Could you check a few things on this model? Use its own coordinates, in mm. Face numbers are marked on the shaded views. A direction names the side the tool comes from. Coordinates: 2 decimals unless noted, no trailing zeros. Loops run counter-clockwise (first coordinate to the right, second up) from the corner with the lowest first, then second, coordinate; pieces in that order, holes last.
1) Thinking about a two-plate mould opening in X: for the marked faces 1, 2 and 3, which applies, released by +X, released by -X, zero draft, split by the parting line, or undercut?
2) Imagine slicing it at B-B on x = 0. Please give me the cut outline in (y, z) (3 decimals), plus the area to 3 significant figures.
3) Imagine slicing it at D-D on z = -2.75. Please give me the cut outline in (x, y) (3 decimals).
4) Imagine slicing it at C-C on y = 7. Please give me the cut outline in (x, z), plus the area to 3 significant figures.
5) For the marked faces 4 and 5, which set-ups out of +Z, -Z, +X, -X, +Y, -Y let a thin tool reach every point of the face, with its end or its side?
6) If I drill on line 1 along Y through (x, z) = (0, -8.75) (3 decimals); line 2 along X through (y, z) = (8.5, -3); line 3 along Y through (x, z) = (1, -2.5), over which ranges is the centre line in solid material (lowest first)?
7) Will these pins go through, and if not, where does the flat tip stop? P1, Ø11.5, axis at x = 0, y = 0, coming from the -Z side; P2, Ø3, axis at y = 6.5, z = -3.5, coming from the -X side; P3, Ø2, axis at y = 5.5, z = -6, coming from the +X side; P4, Ø6, axis at y = 4.5, z = -6, coming from the +X side.
8) Imagine slicing it at A-A on y = 0. Please give me the cut outline in (x, z) (3 decimals).
```python
from build123d import *

# Parameters (mm, degrees)
CROQUIS1_W            = 14.288
CROQUIS1_H            = 15.875
CORTAR_EXTRUIR1_REACH = 28.612
CROQUIS2_R            = 9.525
CROQUIS3_W            = 3.96875
CROQUIS3_H            = 15.875


with BuildPart() as part:
    # Croquis1 → Revolución1 (revolve)
    with BuildSketch(Plane(origin=(0, 0, 0), x_dir=(0, 0, -1), z_dir=(1, 0, 0)), mode=Mode.PRIVATE) as revoluci_n1_sk:
        with Locations((7.144, 7.9375)):
            Rectangle(CROQUIS1_W, CROQUIS1_H)
    revolve(revoluci_n1_sk.sketch.rotate(Axis((0, 0, 0), (0, 0, -1)), 90), axis=Axis((0, 0, 0), (0, 0, -1)))

    # Croquis2 → Cortar-Extruir1 (cut, up to next)
    with BuildSketch(Plane.XY, mode=Mode.PRIVATE) as cortar_extruir1_sk1:
        Circle(CROQUIS2_R)
    cortar_extruir1_tool1 = extrude(cortar_extruir1_sk1.sketch, amount=-CORTAR_EXTRUIR1_REACH, mode=Mode.PRIVATE) & part.part
    add(cortar_extruir1_tool1.solids().sort_by_distance((0, 0, 0))[0], mode=Mode.SUBTRACT)

    # Croquis3 → Taladro roscado 1/8-27 NPSM1 (revolve, cut)
    with BuildSketch(Plane(origin=(15.875, 0, -7.144), x_dir=(0, 0, -1), z_dir=(0, 1, 0))):
        with Locations((1.984375, 7.9375)):
            Rectangle(CROQUIS3_W, CROQUIS3_H)
    revolve(axis=Axis((22.225, 0, -7.144), (-1, 0, 0)), mode=Mode.SUBTRACT)


solid = part.part
```
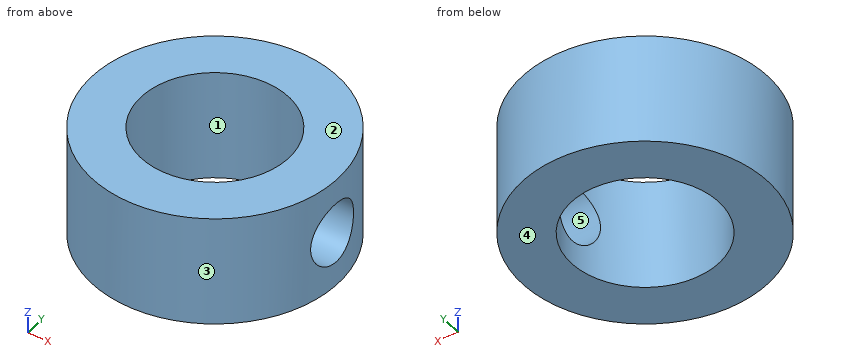
Filled in:
1. face 1: undercut
1. face 2: zero draft
1. face 3: split by the parting line
2. outline: (-15.875, -14.288) - (-9.525, -14.288) - (-9.525, 0) - (-15.875, 0) - close; (9.525, -14.288) - (15.875, -14.288) - (15.875, 0) - (9.525, 0) - close
2. area: 181 mm2
3. outline: circle Ø31.75 at (0, 0); hole circle Ø19.05 at (0, 0)
4. outline: (-14.25, -14.29) - (-6.46, -14.29) - (-6.46, 0) - (-14.25, 0) - close; (6.46, -14.29) - (14.25, -14.29) - (14.25, 0) - (6.46, 0) - close
4. area: 223 mm2
5. face 4: -Z, +X, -X, +Y, -Y
5. face 5: +X
6. line 1: y = -15.875 to -9.525, 9.525 to 15.875
6. line 2: x = -13.41 to -4.3, 4.3 to 13.41
6. line 3: y = -15.84 to -9.47, 9.47 to 15.84
7. P1: passes through
7. P2: stops at x = -15.07
7. P3: stops at x = 15.22
7. P4: stops at x = 15.7
8. outline: (-15.875, -14.288) - (-9.525, -14.288) - (-9.525, 0) - (-15.875, 0) - close; (9.525, -14.288) - (15.875, -14.288) - (15.875, -11.113) - (9.525, -11.113) - close; (9.525, -3.175) - (15.875, -3.175) - (15.875, 0) - (9.525, 0) - close
